Design review of the part shown in the three views and the two pictorial views. Dimensions are in mm from the part's minimum x, y and z. A direction names the side the tool comes from. Give positions to 0.01 mm unless a question says otherwise; leave off trailing zeros. Order: outer loops, then holes, each group sorted by start corner. A loop starts at its lowest first (then second) coordinate and runs counter-clockwise, first axis right, second up. Notation, with made-up numbers: M 59,49 L 64,49 A35 ccw 64,84 Z; hole C 40.25,7.25 d10. An arc over 180 degrees is marked long. Answer as a JSON object with one key per item and string values.
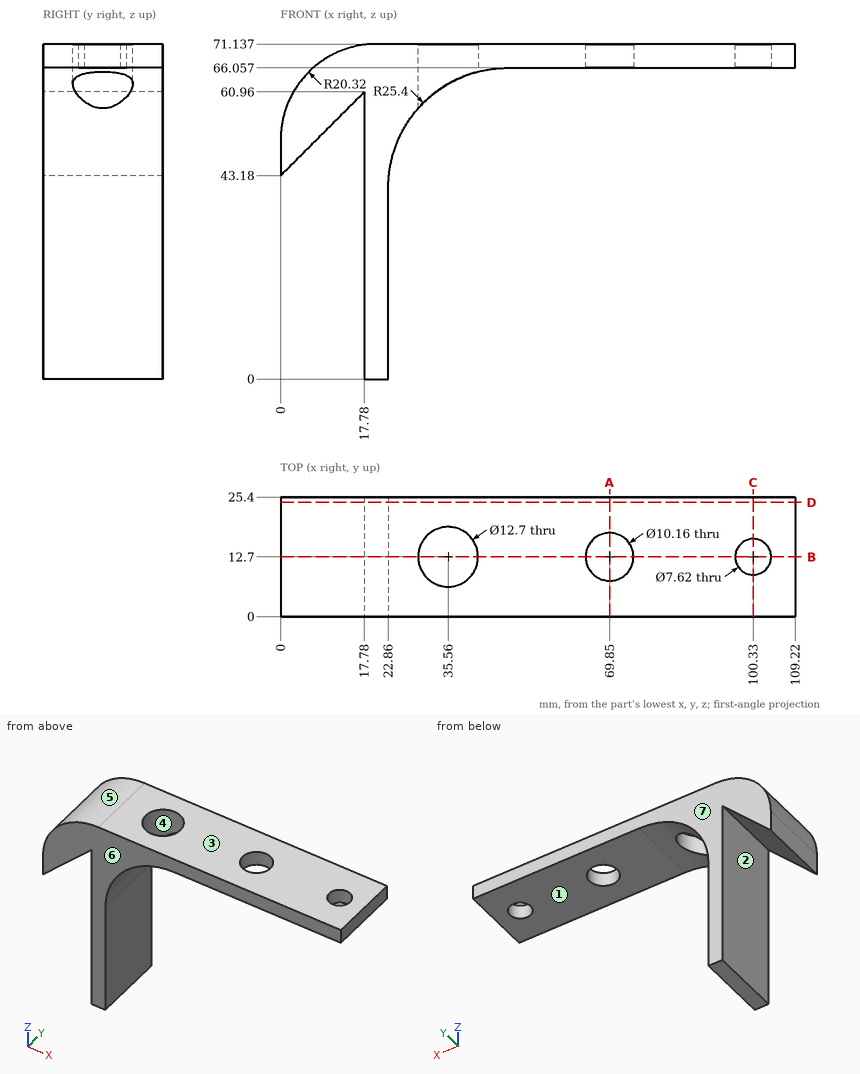
(1) To check wall thickness, follow L1, parallel to Y at x = 35, z = 64 (1 decimal); L2, parallel to Y at x = 69.85, z = 69.8; L3, parallel to Z at x = 54, y = 10.5. State the ranges of each line that lie inside material, in increasing order. Write a range as from..to.
Checked values:
{"L1": "y = 0..6.4, 19..25.4", "L2": "y = 0..7.62, 17.78..25.4", "L3": "z = 66.06..71.14"}
(2) We need section A-A (x = 69.85). Write out the cut boundary in (y, z).
Checked values:
{"outline": "M 0,66.06 L 7.62,66.06 L 7.62,71.14 L 0,71.14 Z; M 17.78,66.06 L 25.4,66.06 L 25.4,71.14 L 17.78,71.14 Z"}
(3) Insertion check: pin 1 (7.5 mm diameter, centred on x = 72.5, y = 7.5, fed in from -Z); pin 2 (12.5 mm diameter, centred on y = 11, z = 21.5, fed in from -X); pin 3 (1.5 mm diameter, centred on y = 15.5, z = 52.5, fed in from -X). Each pin has a flat end and moves straight along its axis. Give the tip position at first contact, or say it passes through.
Checked values:
{"pin 1": "stops at z = 66.06", "pin 2": "stops at x = 17.78", "pin 3": "stops at x = 0.02"}
(4) We need section C-C (x = 100.33). Write out the cut boundary in (y, z).
Checked values:
{"outline": "M 0,66.06 L 8.89,66.06 L 8.89,71.14 L 0,71.14 Z; M 16.51,66.06 L 25.4,66.06 L 25.4,71.14 L 16.51,71.14 Z"}
(5) We need section B-B (y = 12.7). Write out the cut boundary in (x, z).
Checked values:
{"outline": "M 0,43.18 L 17.78,60.96 L 17.78,0 L 22.86,0 L 22.86,40.66 A25.4 cw 29.21,57.46 L 29.21,71.14 L 20.32,71.14 A20.32 ccw 0,50.82 Z; M 41.91,65.25 A25.4 cw 48.26,66.06 L 64.77,66.06 L 64.77,71.14 L 41.91,71.14 Z; M 74.93,66.06 L 96.52,66.06 L 96.52,71.14 L 74.93,71.14 Z; M 104.14,66.06 L 109.22,66.06 L 109.22,71.14 L 104.14,71.14 Z"}
(6) Draft analysis for pull direction Y (two halves, no side actions). For the marked faces 4, 5, 6 and 7, state which applies: +Y half, -Y half, draft (parallel to the pull), parting line (faces both ways), or undercut.
Checked values:
{"face 4": "undercut", "face 5": "draft", "face 6": "-Y half", "face 7": "+Y half"}
(7) Tool access review of the marked faces 1, 2 and 3: name each direction out of +Z, -Z, +X, -X, +Y, -Y from which nothing blocks a thin tool from reaching the whole face with its end or side.
Checked values:
{"face 1": "-Z, +X, +Y, -Y", "face 2": "-Z, +Y, -Y", "face 3": "+Z, +X, -X, +Y, -Y"}
(8) We need section D-D (y = 24.25). Write out the cut boundary in (x, z), plus the area to 3 significant figures.
Checked values:
{"outline": "M 0,43.18 L 17.78,60.96 L 17.78,0 L 22.86,0 L 22.86,40.66 A25.4 cw 48.26,66.06 L 109.22,66.06 L 109.22,71.14 L 20.32,71.14 A20.32 ccw 0,50.82 Z", "area": "1,190 mm^2"}
